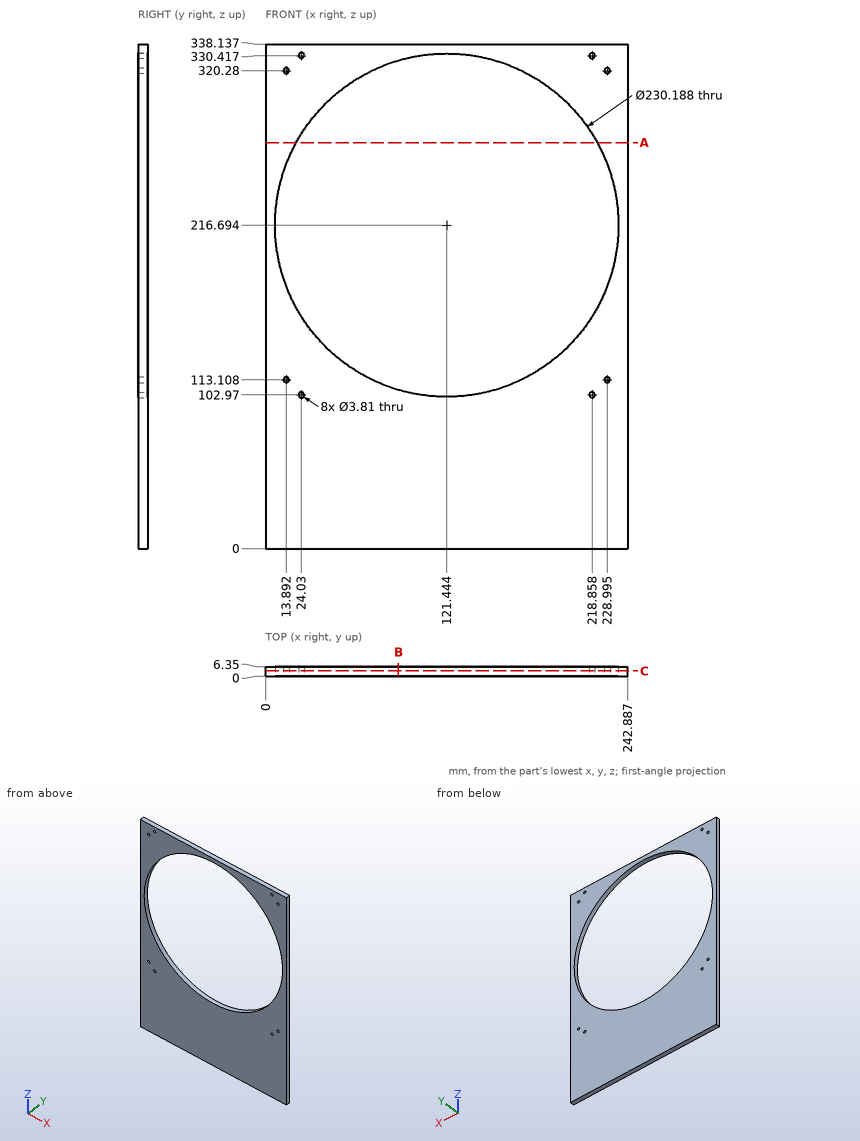
Here's the drawing with two shaded views (mm, measured from the low corner). I have some questions. Give positions to 0.01 mm unless a question says otherwise; leave off trailing zeros. Write each loop counter-clockwise with the first axis right and the second up, starting at its lowest first coordinate (ties: lowest second). Pieces come first, ordered by that corner, then holes. Notation, with made-up numbers: (-23.5, -4.75) -> (19.5, -4.75) arc R27 ccw to (19.5, 24.25) -> close; hole circle Ø5 at (10, 33.5). An arc over 180 degrees is marked (long way). Answer as a JSON object with one key per item and string values. Group by question number.
Item 1: Suppose I cut it at A-A (z = 272). Please give me the cut outline in (x, y).
Item 2: Suppose I cut it at B-B (x = 89). Please give me the cut outline in (y, z).
Item 3: Please list where these lines run through material, in increasing order: line 1 (Z direction, x = 32, y = 4) (1 decimal); line 2 (Z direction, x = 219, y = 5) (1 decimal); line 3 (X direction, y = 2.25, z = 223.5) (1 decimal). Write a range as [from, to].
Item 4: Suppose I cut it at C-C (y = 3.5). State how many separate pieces and enclosed holes the cut face has, plus the area to 3 significant figures.
Findings:
{
 "1": {"outline": "(0, 0) -> (20.51, 0) -> (20.51, 6.35) -> (0, 6.35) -> close; (222.38, 0) -> (242.89, 0) -> (242.89, 6.35) -> (222.38, 6.35) -> close"},
 "2": {"outline": "(0, 0) -> (6.35, 0) -> (6.35, 106.27) -> (0, 106.27) -> close; (0, 327.12) -> (6.35, 327.12) -> (6.35, 338.14) -> (0, 338.14) -> close"},
 "3": {"line 1": "z = [0, 144.3], [289.1, 338.1]", "line 2": "z = [0, 101.1], [104.9, 155.6], [277.8, 328.5], [332.3, 338.1]", "line 3": "x = [0, 6.6], [236.3, 242.9]"},
 "4": {"separate pieces": "1", "enclosed holes": "9", "area": "40,400 mm²"}
}
